from build123d import *

# Parameters (mm, degrees)
CUT_EXTRUDE1_DEPTH = 2.5


with BuildPart() as part:
    # Sketch1 → Revolve1 (revolve)
    with BuildSketch(Plane.XY):
        Polygon((0, 0), (-25, 0), (-25, 1.75), (-24.65, 2.1), (0, 2.1), (0, 4.6), (3.75, 4.6), (4, 4.35), (4, 0), align=None)
    revolve(axis=Axis((0, 0, 0), (-1, 0, 0)))

    # Sketch2 → Cut-Extrude1 (cut)
    with BuildSketch(Plane(origin=(4, 0, 0), x_dir=(0, 0, -1), z_dir=(1, 0, 0))):
        Polygon((0, 2.75), (-1.58771324, 2.75), (-2.38156986, 1.375), (-3.175426481, 0), (-2.38156986, -1.375), (-1.58771324, -2.75), (0, -2.75), (1.58771324, -2.75), (2.38156986, -1.375), (3.175426481, 0), (2.38156986, 1.375), (1.58771324, 2.75), align=None)
    extrude(amount=-CUT_EXTRUDE1_DEPTH, mode=Mode.SUBTRACT)


solid = part.part
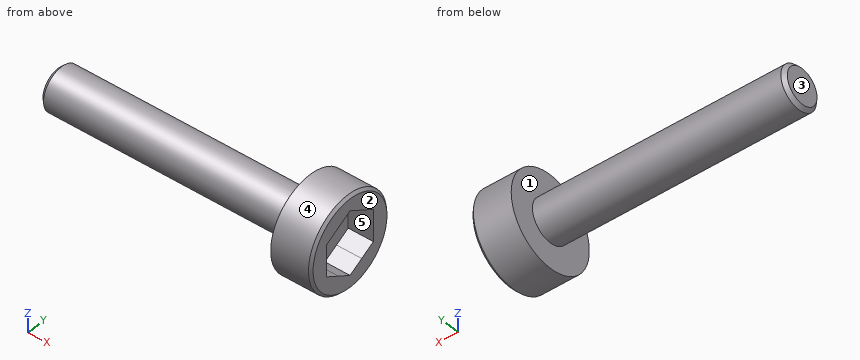
Design review of the part built by this model. Coordinates are the model's own, in mm. Face numbers are marked on the shaded views. A direction names the side the tool comes from. Round coordinates to 2 decimals unless told otherwise and drop trailing zeros. Order: outer loops, then holes, each group sorted by start corner. A loop starts at its lowest first (then second) coordinate and runs counter-clockwise, first axis right, second up. Notation, with made-up numbers: M 40,67.5 L 44,67.5 A17 cw 44,84.5 Z; hole C 0.5,58 d9. An arc over 180 degrees is marked long. Answer as CSV lines item,"result". Start each with the question number.
1) Wall thickness on line 1 along X through (y, z) = (0.75, 2); line 2 along Z through (x, y) = (0.25, -0.25); line 3 along X through (y, z) = (0.75, 0.5): over which ranges is each line inside the solid? List them lowest first. Write a range as [from, to].
2) The part is to be moulded in two halves that separate along Y. For the marked faces 3, 4 and 5, say which applies: +Y half, -Y half, draft (parallel to the pull), parting line (faces both ways), or undercut.
3) Tool access review of the marked faces 1 and 2: name each direction out of +Z, -Z, +X, -X, +Y, -Y from which nothing blocks a thin tool from reaching the whole face with its end or side.
4) Add section B-B (x = -7.5). Give the boundary of the cut face in (y, z), then the cut area to 3 significant figures.
5) For pin 1 Ø3 at (x, z) = (2.5, -0.5) entering from -Y; pin 2 Ø2 at (x, z) = (-10.5, 1.5) entering from -Y; pin 3 Ø2 at (x, y) = (-7, -2) entering from +Z; pin 4 Ø4.5 at (y, z) = (0, 0) entering from +X, all flat-tipped, find the tip position at first contact; note any pin that passes through.
6) Add section A-A (z = 0). Give the boundary of the cut face in (x, y), then the cut area to 3 significant figures.
Resolved:
1,line 1,"[0, 1.5]"
1,line 2,"[-4.59, 4.59]"
1,line 3,"[-25, 1.5]"
2,face 3,"draft"
2,face 4,"parting line"
2,face 5,"undercut"
3,face 1,"-X"
3,face 2,"+Z, -Z, +X, +Y, -Y"
4,outline,"C 0,0 d4.2"
4,area,"13.9 mm^2"
5,pin 1,"y = -4.6"
5,pin 2,"y = -2.04"
5,pin 3,"z = 1.85"
5,pin 4,"x = 1.5"
6,outline,"M -25,-1.75 L -24.65,-2.1 L 0,-2.1 L 0,-4.6 L 3.75,-4.6 L 4,-4.35 L 4,-2.75 L 1.5,-2.75 L 1.5,2.75 L 4,2.75 L 4,4.35 L 3.75,4.6 L 0,4.6 L 0,2.1 L -24.65,2.1 L -25,1.75 Z"
6,area,"128 mm^2"
